The model under review builds one solid part; all positions refer to its coordinate system, in mm. Face numbers are marked on the shaded views. Round coordinates to 2 decimals unless told otherwise and drop trailing zeros. Loops run counter-clockwise (first coordinate to the right, second up) from the corner with the lowest first, then second, coordinate; pieces in that order, holes last. Notation, with made-up numbers: M 46,-33 L 89,-33 A19 cw 89,-21 Z; hole C 13.5,5.5 d3. An arc over 180 degrees is marked long. Return JSON: item names as keys, results as strings. Group by question number.
Q1. Consider section A-A (z = 4.25). State the section outline as (x, y) points (3 decimals).
Q2. To check wall thickness, follow line 1 along Y through (x, z) = (-0.5, 3.5); line 2 along X through (y, z) = (25, 3.5) (3 decimals); line 3 along Y through (x, z) = (-10, 6.75). State the ranges of each line that lie inside material, in increasing order.
Q3. Draft analysis for pull direction Y (two halves, no side actions). For the marked faces 1, 2 and 3, state which applies: pulls with the +Y half, pulls with the -Y half, needs draft (parallel to the pull), parting line crosses it, or undercut.
Q4. Consider section B-B (x = 0). Count the separate pieces of the cut face and the enclosed holes in it, and give its area (3 significant figures).
Q5. Clearance check with flat-ended pins moving along their axes: pin 1 Ø1.5 at (x, z) = (16, 1.5) entering from -Y; pin 2 Ø1 at (y, z) = (33, 4.5) entering from +X; pin 3 Ø1.5 at (x, z) = (-9, 1.5) entering from -Y. State where each tip first meets the part, or that it passes through.
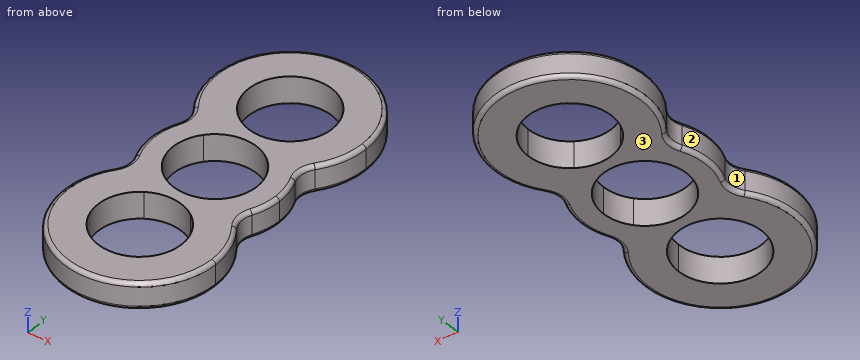
from build123d import *

# Parameters (mm, degrees)
F1_DEPTH = 7
F2_R     = 1


# Not quite as in the source:
# - a feature names something its author has since deleted; it is built from what else it names


with BuildPart() as f1:
    # F0 (on Top) → F1 (new body)
    with BuildSketch(Plane.XY):
        with BuildLine():
            ThreePointArc((8.5900351571, 6.911), (10.3984557172, 3.6637062787), (11.025, 0))
            ThreePointArc((11.025, 0), (10.3984557172, -3.6637062787), (8.5900351571, -6.911))
            ThreePointArc((8.5900351571, -6.911), (11.2087291798, -8.4058740762), (13.5732787491, -10.277))
            ThreePointArc((13.5732787491, -10.277), (14.5991765239, -8.7586911022), (15.455952476, -7.1389185498))
            ThreePointArc((15.455952476, -7.1389185498), (16.628111978, -3.6546568989), (17.025, 0))
            ThreePointArc((17.025, 0), (16.628111978, 3.6546568989), (15.455952476, 7.1389185498))
            ThreePointArc((15.455952476, 7.1389185498), (14.5991765239, 8.7586911022), (13.5732787491, 10.277))
            ThreePointArc((13.5732787491, 10.277), (11.2087291798, 8.4058740762), (8.5900351571, 6.911))
        make_face()
        with BuildLine():
            ThreePointArc((-8.5900351571, -6.911), (-11.025, 0), (-8.5900351571, 6.911))
            ThreePointArc((-8.5900351571, 6.911), (-11.2087291798, 8.4058740762), (-13.5732787491, 10.277))
            ThreePointArc((-13.5732787491, 10.277), (-14.5991765239, 8.7586911022), (-15.455952476, 7.1389185498))
            ThreePointArc((-15.455952476, 7.1389185498), (-17.025, 0), (-15.455952476, -7.1389185498))
            ThreePointArc((-15.455952476, -7.1389185498), (-14.5991765239, -8.7586911022), (-13.5732787491, -10.277))
            ThreePointArc((-13.5732787491, -10.277), (-11.2087291798, -8.4058740762), (-8.5900351571, -6.911))
        make_face()
        with BuildLine():
            ThreePointArc((6.1741937935, 15.866), (10.2615738659, 13.584944858), (13.5732787491, 10.277))
            ThreePointArc((13.5732787491, 10.277), (14.88595909, 11.6056412259), (16.0691422874, 13.0508037447))
            ThreePointArc((16.0691422874, 13.0508037447), (19.0103287623, 18.7065092876), (20.025, 25))
            ThreePointArc((20.025, 25), (-6.2934907124, 44.0103287623), (-16.0691422874, 13.0508037447))
            ThreePointArc((-16.0691422874, 13.0508037447), (-14.88595909, 11.6056412259), (-13.5732787491, 10.277))
            ThreePointArc((-13.5732787491, 10.277), (-10.2615738659, 13.584944858), (-6.1741937935, 15.866))
            ThreePointArc((-6.1741937935, 15.866), (-5.1710800819, 34.737071212), (11.025, 25))
            ThreePointArc((11.025, 25), (9.737071212, 19.8289199181), (6.1741937935, 15.866))
        make_face()
        with BuildLine():
            ThreePointArc((16.0691422874, 13.0508037447), (14.88595909, 11.6056412259), (13.5732787491, 10.277))
            ThreePointArc((13.5732787491, 10.277), (14.5991765239, 8.7586911022), (15.455952476, 7.1389185498))
            ThreePointArc((15.455952476, 7.1389185498), (14.9507513772, 10.1790618755), (16.0691422874, 13.0508037447))
        make_face()
        with BuildLine():
            ThreePointArc((16.0691422874, -13.0508037447), (14.88595909, -11.6056412259), (13.5732787491, -10.277))
            ThreePointArc((13.5732787491, -10.277), (10.2615738659, -13.584944858), (6.1741937935, -15.866))
            ThreePointArc((6.1741937935, -15.866), (9.737071212, -19.8289199181), (11.025, -25))
            ThreePointArc((11.025, -25), (-5.1710800819, -34.737071212), (-6.1741937935, -15.866))
            ThreePointArc((-6.1741937935, -15.866), (-10.2615738659, -13.584944858), (-13.5732787491, -10.277))
            ThreePointArc((-13.5732787491, -10.277), (-14.88595909, -11.6056412259), (-16.0691422874, -13.0508037447))
            ThreePointArc((-16.0691422874, -13.0508037447), (-6.2934907124, -44.0103287623), (20.025, -25))
            ThreePointArc((20.025, -25), (19.0103287623, -18.7065092876), (16.0691422874, -13.0508037447))
        make_face()
        with BuildLine():
            ThreePointArc((15.455952476, -7.1389185498), (14.5991765239, -8.7586911022), (13.5732787491, -10.277))
            ThreePointArc((13.5732787491, -10.277), (14.88595909, -11.6056412259), (16.0691422874, -13.0508037447))
            ThreePointArc((16.0691422874, -13.0508037447), (14.9507513772, -10.1790618755), (15.455952476, -7.1389185498))
        make_face()
        with BuildLine():
            ThreePointArc((-15.455952476, 7.1389185498), (-14.5991765239, 8.7586911022), (-13.5732787491, 10.277))
            ThreePointArc((-13.5732787491, 10.277), (-14.88595909, 11.6056412259), (-16.0691422874, 13.0508037447))
            ThreePointArc((-16.0691422874, 13.0508037447), (-14.9507513772, 10.1790618755), (-15.455952476, 7.1389185498))
        make_face()
        with BuildLine():
            ThreePointArc((-16.0691422874, -13.0508037447), (-14.88595909, -11.6056412259), (-13.5732787491, -10.277))
            ThreePointArc((-13.5732787491, -10.277), (-14.5991765239, -8.7586911022), (-15.455952476, -7.1389185498))
            ThreePointArc((-15.455952476, -7.1389185498), (-14.9507513772, -10.1790618755), (-16.0691422874, -13.0508037447))
        make_face()
        with BuildLine():
            ThreePointArc((-8.5900351571, 6.911), (0, 11.025), (8.5900351571, 6.911))
            ThreePointArc((8.5900351571, 6.911), (11.2087291798, 8.4058740762), (13.5732787491, 10.277))
            ThreePointArc((13.5732787491, 10.277), (10.2615738659, 13.584944858), (6.1741937935, 15.866))
            ThreePointArc((6.1741937935, 15.866), (0, 13.975), (-6.1741937935, 15.866))
            ThreePointArc((-6.1741937935, 15.866), (-10.2615738659, 13.584944858), (-13.5732787491, 10.277))
            ThreePointArc((-13.5732787491, 10.277), (-11.2087291798, 8.4058740762), (-8.5900351571, 6.911))
        make_face()
        with BuildLine():
            ThreePointArc((13.5732787491, -10.277), (11.2087291798, -8.4058740762), (8.5900351571, -6.911))
            ThreePointArc((8.5900351571, -6.911), (0, -11.025), (-8.5900351571, -6.911))
            ThreePointArc((-8.5900351571, -6.911), (-11.2087291798, -8.4058740762), (-13.5732787491, -10.277))
            ThreePointArc((-13.5732787491, -10.277), (-10.2615738659, -13.584944858), (-6.1741937935, -15.866))
            ThreePointArc((-6.1741937935, -15.866), (0, -13.975), (6.1741937935, -15.866))
            ThreePointArc((6.1741937935, -15.866), (10.2615738659, -13.584944858), (13.5732787491, -10.277))
        make_face()
    extrude(amount=F1_DEPTH)

    # F2
    f2_edges = [f1.edges().sort_by_distance(p)[0] for p in [
        (16.069142, 13.050804, 3.5),
        (-16.069142, 13.050804, 3.5),
        (0, 45.025, 0),
        (0, 45.025, 7),
        (-15.455952, 7.138919, 3.5),
        (-14.950751, 10.179062, 0),
        (-14.950751, 10.179062, 7),
        (-15.455952, -7.138919, 3.5),
        (-16.069142, -13.050804, 3.5),
        (-14.950751, -10.179062, 0),
        (-14.950751, -10.179062, 7),
        (16.069142, -13.050804, 3.5),
        (0, -45.025, 0),
        (0, -45.025, 7),
    ]]
    fillet(f2_edges, radius=F2_R)


solid = f1.part
Values:
{
 "1": {"outline": "M -16.069,-13.051 A20.025 ccw long 16.069,-13.051 A5.819 cw 15.456,-7.139 A17.025 ccw 15.456,7.139 A5.819 cw 16.069,13.051 A20.025 ccw long -16.069,13.051 A5.819 cw -15.456,7.139 A17.025 ccw -15.456,-7.139 A5.819 cw Z; hole C 0,-25 d22.05; hole C 0,0 d22.05; hole C 0,25 d22.05"},
 "2": {"line 1": "y = -45.02 to -36.01, -13.99 to -11.01, 11.01 to 13.99, 36.01 to 45.02", "line 2": "x = -20.025 to -11.025, 11.025 to 20.025", "line 3": "y = -41.96 to -29.64, -20.36 to -4.64, 4.64 to 20.36, 29.64 to 41.96"},
 "3": {"face 1": "undercut", "face 2": "undercut", "face 3": "needs draft"},
 "4": {"separate pieces": "4", "enclosed holes": "0", "area": "166 mm2"},
 "5": {"pin 1": "stops at y = -37.98", "pin 2": "stops at x = 18.57", "pin 3": "stops at y = -43.25"}
}
